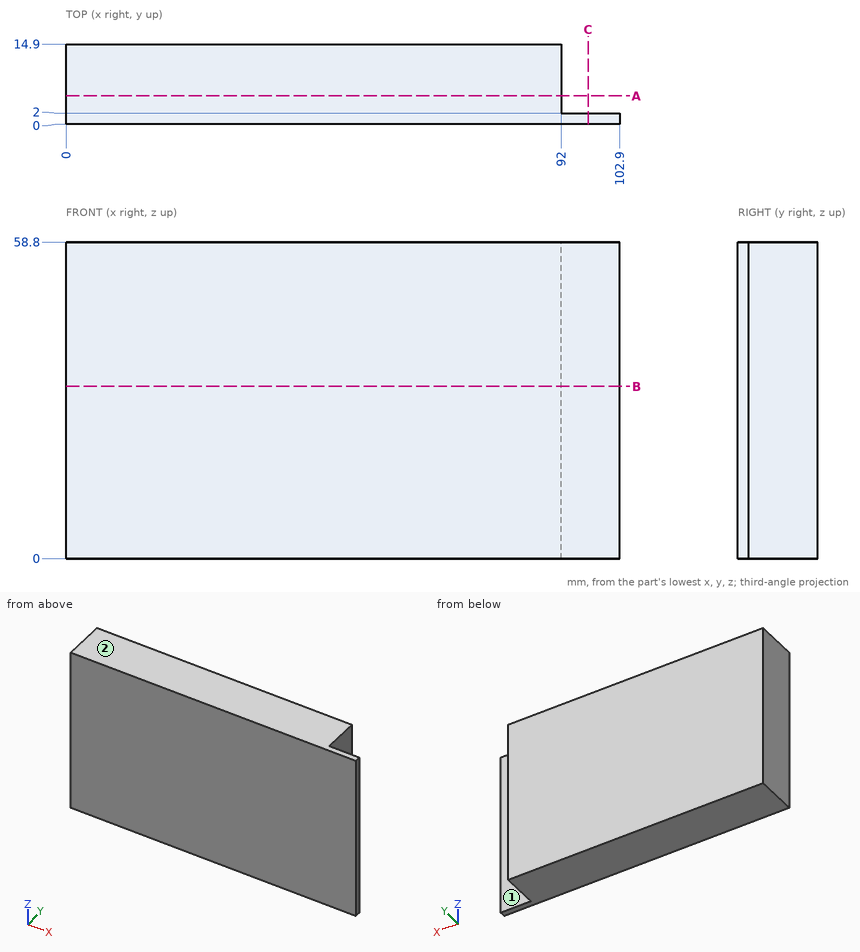
Print and shaded views of the part. All mm, measured from the part's lowest x, y and z. A direction names the side the tool comes from. Round coordinates to 2 decimals unless told otherwise and drop trailing zeros. Write each loop counter-clockwise with the first axis right and the second up, starting at its lowest first coordinate (ties: lowest second). Pieces come first, ordered by that corner, then holes. Notation, with made-up numbers: M 69.5,40 L 93.5,40 A31 cw 93.5,69 Z; hole C 1.25,-9.75 d6. An arc over 180 degrees is marked long. One line per question, with ' | ' between items.
(1) Saw through at A-A on y = 5.25. Write the cut outline in (x, z), then the cut area to 3 significant figures.
Answer key:
outline: M 0,0 L 92,0 L 92,58.8 L 0,58.8 Z | area: 5,410 mm^2
(2) Pin check, flat tip, straight feed: pin 1 (6.5 mm diameter, centred on y = 8.5, z = 33, fed in from +X). Stop position of the tip, or through.
Answer key:
pin 1: stops at x = 92
(3) 3-axis set-ups, long thin cutter, end or side, ignore diameter. For the marked faces 1 and 2: which of +Z, -Z, +X, -X, +Y, -Y reach the whole face in a straight line?
Answer key:
face 1: +Z, -Z, +X, +Y | face 2: +Z, +X, -X, +Y, -Y
(4) Saw through at C-C on x = 97. Write the cut outline in (y, z), then the cut area to 3 significant figures.
Answer key:
outline: M 0,0 L 2,0 L 2,58.8 L 0,58.8 Z | area: 118 mm^2
(5) Probe line 1 along X through (y, z) = (8.5, 24.5). List the from-to ranges inside material, lowest first.
Answer key:
line 1: x = 0 to 92
(6) Saw through at B-B on z = 32. Write the cut outline in (x, y), then the cut area to 3 significant figures.
Answer key:
outline: M 0,0 L 102.9,0 L 102.9,2 L 92,2 L 92,14.9 L 0,14.9 Z | area: 1,390 mm^2
